Build history of the part. All positions in model axes, mm. A direction names the side the tool comes from. Round coordinates to 2 decimals unless told otherwise and drop trailing zeros. Loops run counter-clockwise (first coordinate to the right, second up) from the corner with the lowest first, then second, coordinate; pieces in that order, holes last. Notation, with made-up numbers: (51.5, 65) - (91.5, 65) arc R20 cw to (91.5, 75) - close; hole circle Ø9 at (-4.75, 37.25). An arc over 180 degrees is marked (long way). One line per question, with ' | ' between items. Start each with the question number.
from build123d import *

# Parameters (mm, degrees)
BOSS_EXTRUDE1_DEPTH = 20
SKETCH2_W           = 20
SKETCH2_H           = 20
CUT_EXTRUDE1_DEPTH  = 10
SKETCH3_W           = 10
SKETCH3_H           = 10
CUT_EXTRUDE2_DEPTH  = 194
BOSS_EXTRUDE3_DEPTH = 15
SKETCH6_W           = 30
SKETCH6_H           = 30
BOSS_EXTRUDE4_DEPTH = 20
SKETCH7_W           = 20
SKETCH7_H           = 20
CUT_EXTRUDE3_DEPTH  = 10
SKETCH8_W           = 10
SKETCH8_H           = 10
CUT_EXTRUDE4_DEPTH  = 41
BOSS_EXTRUDE7_DEPTH = 20
BOSS_EXTRUDE8_DEPTH = 15
SKETCH12_W          = 20
SKETCH12_H          = 20
CUT_EXTRUDE5_DEPTH  = 10
SKETCH13_W          = 10
SKETCH13_H          = 10
CUT_EXTRUDE6_DEPTH  = 31


with BuildPart() as part:
    # Sketch1 → Boss-Extrude1 (new body)
    with BuildSketch(Plane.XY):
        Polygon((-40, 0), (-40, 30), (-30, 40), (-10, 40), (0, 30), (0, 0), (-10, -10), (-30, -10), align=None)
    extrude(amount=BOSS_EXTRUDE1_DEPTH)

    # Sketch2 → Cut-Extrude1 (cut)
    with BuildSketch(Plane.XY.offset(20)):
        with Locations((-30, 15)):
            Rectangle(SKETCH2_W, SKETCH2_H)
    extrude(amount=-CUT_EXTRUDE1_DEPTH, mode=Mode.SUBTRACT)

    # Sketch3 → Cut-Extrude2 (cut)
    with BuildSketch(Plane.XY.offset(10)):
        with Locations((-30, 15)):
            Rectangle(SKETCH3_W, SKETCH3_H)
    extrude(amount=-CUT_EXTRUDE2_DEPTH, mode=Mode.SUBTRACT)

    # Sketch5 → Boss-Extrude3 (add)
    with BuildSketch(Plane(origin=(0, 0, 0), x_dir=(-1, 0, 0), z_dir=(0, 0, -1))):
        Polygon((30, -10), (25, -15), (15, -15), (10, -10), align=None)
        Polygon((30, 40), (25, 45), (15, 45), (10, 40), align=None)
    extrude(amount=-BOSS_EXTRUDE3_DEPTH)

    # Sketch6 → Boss-Extrude4 (add)
    with BuildSketch(Plane.XY.offset(20)):
        with Locations((10, 15)):
            Rectangle(SKETCH6_W, SKETCH6_H)
    extrude(amount=BOSS_EXTRUDE4_DEPTH)

    # Sketch7 → Cut-Extrude3 (cut)
    with BuildSketch(Plane.XY.offset(40)):
        with Locations((10, 15)):
            Rectangle(SKETCH7_W, SKETCH7_H)
    extrude(amount=-CUT_EXTRUDE3_DEPTH, mode=Mode.SUBTRACT)

    # Sketch8 → Cut-Extrude4 (cut)
    with BuildSketch(Plane.XY.offset(30)):
        with Locations((10, 15)):
            Rectangle(SKETCH8_W, SKETCH8_H)
    extrude(amount=-CUT_EXTRUDE4_DEPTH, mode=Mode.SUBTRACT)

    # Sketch10 → Boss-Extrude7 (add)
    with BuildSketch(Plane(origin=(0, 0, 20), x_dir=(-1, 0, 0), z_dir=(0, 0, -1))):
        Polygon((-20, 30), (-30, 40), (-50, 40), (-60, 30), (-60, 0), (-50, -10), (-30, -10), (-20, 0), align=None)
    extrude(amount=BOSS_EXTRUDE7_DEPTH)

    # Sketch11 → Boss-Extrude8 (add)
    with BuildSketch(Plane(origin=(0, 0, 0), x_dir=(-1, 0, 0), z_dir=(0, 0, -1))):
        Polygon((-35, 45), (-45, 45), (-50, 40), (-30, 40), align=None)
        Polygon((-50, -10), (-30, -10), (-35, -15), (-45, -15), align=None)
    extrude(amount=-BOSS_EXTRUDE8_DEPTH)

    # Sketch12 → Cut-Extrude5 (cut)
    with BuildSketch(Plane.XY.offset(20)):
        with Locations((50, 15)):
            Rectangle(SKETCH12_W, SKETCH12_H)
    extrude(amount=-CUT_EXTRUDE5_DEPTH, mode=Mode.SUBTRACT)

    # Sketch13 → Cut-Extrude6 (cut)
    with BuildSketch(Plane.XY.offset(10)):
        with Locations((50, 15)):
            Rectangle(SKETCH13_W, SKETCH13_H)
    extrude(amount=-CUT_EXTRUDE6_DEPTH, mode=Mode.SUBTRACT)


solid = part.part
1) Wall check: line 1 (X direction, y = 35, z = 12.5); line 2 (X direction, y = 21, z = 17.5); line 3 (Y direction, x = -3.5, z = 35). Give the ranges that are in metal, low to high. Write a range as [from, to].
2) Saw through at A-A on z = 3.5. Write the cut outline in (x, y).
3) Tool access for faces 1 (the flat face through (55, 15, 5)), 2 (the flat face through (40, 42, 15)), 3 (the flat face through (-20, 15, 15)), 4 (the flat face through (-20, -12, 15)), 5 (the flat face through (27, 37, 10)): list every direction of +Z, -Z, +X, -X, +Y, -Y with a clear straight run to the whole face (end or side of a thin tool).
4) Saw through at D-D on z = 12.5. Write the cut outline in (x, y), and give its area (3 significant figures).
5) Saw through at B-B on y = -5.5. Write the cut outline in (x, z).
6) Two-plate mould, pull along X, no slides. Class faces 6 (the flat face through (10, 5, 35)), 7 (the flat face through (25, 15, 30)), 8 (the flat face through (40, 45, 7)), 9 (the flat face through (-40, 15, 8)): +X half, -X half, draft (parallel to the pull), parting line (faces both ways), or undercut.
7) Saw through at C-C on x = 11.5. Write the cut outline in (y, z), and give its area (3 significant figures).
8) Drop flat-ended pins along their axis: pin 1 (1.5 mm diameter, centred on x = 38, z = 17.5, fed in from -Y); pin 2 (6 mm diameter, centred on y = 25, z = 33, fed in from -X); pin 3 (20 mm diameter, centred on x = 39.5, y = 10, fed in from +Z). Give the stop position or say it passes through.
Answer key:
1) line 1: [-35, -5], [25, 55] | line 2: [-20, 0], [20, 40] | line 3: [0, 30]
2) outline: (-40, 0) - (-25, -15) - (-15, -15) - (0, 0) - (0, 30) - (-15, 45) - (-25, 45) - (-40, 30) - close; (20, 0) - (35, -15) - (45, -15) - (60, 0) - (60, 30) - (45, 45) - (35, 45) - (20, 30) - close; hole (-35, 10) - (-25, 10) - (-25, 20) - (-35, 20) - close; hole (45, 10) - (55, 10) - (55, 20) - (45, 20) - close
3) face 1: +Z, -Z | face 2: +Z, +X, -X, +Y | face 3: +Z, -X | face 4: +Z, +X, -X, -Y | face 5: +Z, -Z, +Y
4) outline: (-40, 0) - (-25, -15) - (-15, -15) - (0, 0) - (0, 30) - (-15, 45) - (-25, 45) - (-40, 30) - (-40, 25) - (-20, 25) - (-20, 5) - (-40, 5) - close; (20, 0) - (35, -15) - (45, -15) - (60, 0) - (60, 5) - (40, 5) - (40, 25) - (60, 25) - (60, 30) - (45, 45) - (35, 45) - (20, 30) - close | area: 3,100 mm²
5) outline: (-34.5, 0) - (-5.5, 0) - (-5.5, 20) - (-34.5, 20) - close; (25.5, 0) - (54.5, 0) - (54.5, 20) - (25.5, 20) - close
6) face 6: undercut | face 7: +X half | face 8: draft | face 9: -X half
7) outline: (0, 20) - (10, 20) - (10, 30) - (5, 30) - (5, 40) - (0, 40) - close; (20, 20) - (30, 20) - (30, 40) - (25, 40) - (25, 30) - (20, 30) - close | area: 300 mm²
8) pin 1: y = -10 | pin 2: x = -5 | pin 3: z = 20
